```python
from build123d import *

# Parameters (mm, degrees)
SKETCH1_W           = 200
SKETCH1_H           = 17.1
BOSS_EXTRUDE1_DEPTH = 6.35
CUT_EXTRUDE1_REACH  = 8.35
CUT_EXTRUDE2_DEPTH  = 6.35
LPATTERN1_COUNT     = 5
LPATTERN1_PITCH     = 32
CUT_EXTRUDE3_DEPTH  = 6.35
LPATTERN2_COUNT     = 5
LPATTERN2_PITCH     = 32
FILLET1_R           = 10
CUT_EXTRUDE6_REACH  = 8.35
FILLET2_R           = 3
CUT_EXTRUDE7_REACH  = 202
SKETCH6_R           = 2.5
CUT_EXTRUDE8_REACH  = 202
SKETCH7_R           = 2.5


with BuildPart() as part:
    # Sketch1 → Boss-Extrude1 (new body)
    with BuildSketch(Plane(origin=(0, 0, 0), x_dir=(1, 0, 0), z_dir=(0, 1, 0))):
        with Locations((100, 8.55)):
            Rectangle(SKETCH1_W, SKETCH1_H)
    extrude(amount=BOSS_EXTRUDE1_DEPTH)

    # Sketch2 → Cut-Extrude1 (cut, up to next)
    with BuildSketch(Plane(origin=(0, 6.35, 0), x_dir=(1, 0, 0), z_dir=(0, 1, 0)), mode=Mode.PRIVATE) as cut_extrude1_sk1:
        with BuildLine():
            Line((2, 11.05), (8, 11.05))
            Line((8, 11.05), (26.371920214, 14.983515942))
            ThreePointArc((26.371920214, 14.983515942), (29.935888288, 12.666895422), (27.605702097, 9.111782008))
            Line((27.605702097, 9.111782008), (11.75, 8.5))
            Line((11.75, 8.5), (8, 6.05))
            Line((8, 6.05), (2, 6.05))
            Line((2, 6.05), (2, 11.05))
        make_face()
    cut_extrude1_tool1 = extrude(cut_extrude1_sk1.sketch, amount=-CUT_EXTRUDE1_REACH, mode=Mode.PRIVATE) & part.part
    add(cut_extrude1_tool1.solids().sort_by_distance((16.294125, 6.35, -10.477607))[0], mode=Mode.SUBTRACT)

    # Sketch3 → Cut-Extrude2 (cut)
    with BuildSketch(Plane(origin=(0, 6.35, 0), x_dir=(1, 0, 0), z_dir=(0, 1, 0))):
        with BuildLine():
            Line((42.420014497, 2.456597748), (11.75, 8.5))
            Line((11.75, 8.5), (27.605702097, 9.111782008))
            Line((27.605702097, 9.111782008), (43.1379451, 8.396826847))
            ThreePointArc((43.1379451, 8.396826847), (45.978326773, 5.040042176), (42.420014497, 2.456597748))
        make_face()
    cut_extrude2 = extrude(amount=-CUT_EXTRUDE2_DEPTH, mode=Mode.SUBTRACT)

    # LPattern1: Cut-Extrude2 ×5
    with Locations(*[(i * LPATTERN1_PITCH, 0, 0) for i in range(1, LPATTERN1_COUNT)]):
        add(cut_extrude2, mode=Mode.SUBTRACT)

    # Sketch4 → Cut-Extrude3 (cut)
    with BuildSketch(Plane(origin=(0, 6.35, 0), x_dir=(1, 0, 0), z_dir=(0, 1, 0))):
        with BuildLine():
            Line((27.605702097, 9.111782008), (58.394623882, 15.141281248))
            ThreePointArc((58.394623882, 15.141281248), (62.130306809, 12.401680657), (59.095650073, 8.901452547))
            Line((59.095650073, 8.901452547), (42.878228619, 8.408781697))
            Line((42.878228619, 8.408781697), (27.605702097, 9.111782008))
        make_face()
    cut_extrude3 = extrude(amount=-CUT_EXTRUDE3_DEPTH, mode=Mode.SUBTRACT)

    # LPattern2: Cut-Extrude3 ×5
    with Locations(*[(i * LPATTERN2_PITCH, 0, 0) for i in range(1, LPATTERN2_COUNT)]):
        add(cut_extrude3, mode=Mode.SUBTRACT)

    # Fillet1
    fillet1_edges = [part.edges().sort_by_distance(p)[0] for p in [
        (11.75, 3.175, -8.5),
    ]]
    fillet(fillet1_edges, radius=FILLET1_R)

    # Sketch5 → Cut-Extrude6 (cut, up to next)
    with BuildSketch(Plane(origin=(0, 6.35, 0), x_dir=(1, 0, 0), z_dir=(0, 1, 0)), mode=Mode.PRIVATE) as cut_extrude6_sk1:
        Polygon((198, 6.05), (193, 6.05), (172.348389916, 8.453443891), (190.130306809, 12.401680657), (194, 11.05), (198, 11.05), align=None)
    cut_extrude6_tool1 = extrude(cut_extrude6_sk1.sketch, amount=-CUT_EXTRUDE6_REACH, mode=Mode.PRIVATE) & part.part
    add(cut_extrude6_tool1.solids().sort_by_distance((188.45236, 6.35, -8.941649))[0], mode=Mode.SUBTRACT)

    # Fillet2
    fillet2_edges = [part.edges().sort_by_distance(p)[0] for p in [
        (190.130306809, 3.175, -12.401680657),
        (194, 3.175, -11.05),
    ]]
    fillet(fillet2_edges, radius=FILLET2_R)

    # Sketch6 → Cut-Extrude7 (cut, up to next)
    with BuildSketch(Plane(origin=(200, 0, 0), x_dir=(0, 0, -1), z_dir=(1, 0, 0)), mode=Mode.PRIVATE) as cut_extrude7_sk1:
        with Locations((8.55, 3.175)):
            Circle(SKETCH6_R)
    cut_extrude7_tool1 = extrude(cut_extrude7_sk1.sketch, amount=-CUT_EXTRUDE7_REACH, mode=Mode.PRIVATE) & part.part
    add(cut_extrude7_tool1.solids().sort_by_distance((200, 3.175, -8.55))[0], mode=Mode.SUBTRACT)

    # Sketch7 → Cut-Extrude8 (cut, up to next)
    with BuildSketch(Plane.ZY, mode=Mode.PRIVATE) as cut_extrude8_sk1:
        with Locations((-8.55, 3.175)):
            Circle(SKETCH7_R)
    cut_extrude8_tool1 = extrude(cut_extrude8_sk1.sketch, amount=-CUT_EXTRUDE8_REACH, mode=Mode.PRIVATE) & part.part
    add(cut_extrude8_tool1.solids().sort_by_distance((0, 3.175, -8.55))[0], mode=Mode.SUBTRACT)


solid = part.part
```
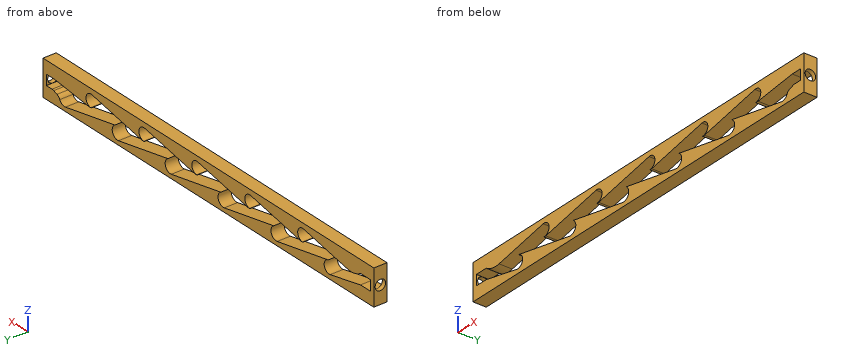
Design review of the part built by this model. Coordinates are the model's own, in mm. Coordinates: 2 decimals unless noted, no trailing zeros. Write each loop counter-clockwise with the first axis right and the second up, starting at its lowest first coordinate (ties: lowest second). Pieces come first, ordered by that corner, then holes.
1) To check wall thickness, follow L1, parallel to Y at x = 199.1, z = -8.55 (3 decimals); L2, parallel to X at y = 5.75, z = -9; L3, parallel to Z at x = 177.5, y = 5.25. State the ranges of each line that lie inside material, in increasing order.
2) Add section B-B (x = 24). Write out the cut boundary in (y, z).
3) Insertion check: pin 1 (1.7 mm diameter, centred on x = 195.5, y = 2.5, fed in from +Z). The pin has a flat end and moves straight along its axis. Give the tip position at first contact, or say it passes through.
4) Add section A-A (x = 53.5). Write out the cut boundary in (y, z).
Check result:
1. L1: y = 0 to 0.675, 5.675 to 6.35
1. L2: x = 0 to 2, 198 to 200
1. L3: z = -17.1 to -13.4, -7.85 to 0
2. outline: (0, -17.1) - (6.35, -17.1) - (6.35, -14.48) - (0, -14.48) - close; (0, -6.09) - (6.35, -6.09) - (6.35, 0) - (0, 0) - close
3. pin 1: stops at z = 0
4. outline: (0, -17.1) - (6.35, -17.1) - (6.35, -14.18) - (0, -14.18) - close; (0, -6.58) - (6.35, -6.58) - (6.35, 0) - (0, 0) - close
